Verification items for the finished model (mm, model axes). Face numbers are marked on the shaded views. Coordinates: 2 decimals unless noted, no trailing zeros. Order: outer loops, then holes, each group sorted by start corner. A loop starts at its lowest first (then second) coordinate and runs counter-clockwise, first axis right, second up. Notation, with made-up numbers: (53, 32.25) -> (104, 32.25) arc R18 cw to (104, 41.25) -> close; hole circle Ø11 at (77.5, 3.25). An arc over 180 degrees is marked (long way). Write item = value, one per line. Start each with the question number.
from build123d import *

# Parameters (mm, degrees)
SKETCH1_R           = 101.6
BOSS_EXTRUDE1_DEPTH = 76.2
SKETCH2_R           = 12.7
BOSS_EXTRUDE2_DEPTH = 609.6


with BuildPart() as part:
    # Sketch1 → Boss-Extrude1 (new body)
    with BuildSketch(Plane.XY):
        Circle(SKETCH1_R)
    boss_extrude1 = extrude(amount=BOSS_EXTRUDE1_DEPTH)

    # Sketch2 → Boss-Extrude2 (add)
    with BuildSketch(Plane.XY.offset(76.2)):
        Circle(SKETCH2_R)
    extrude(amount=BOSS_EXTRUDE2_DEPTH)

    # Mirror1: Boss-Extrude1 across plane
    add(boss_extrude1.mirror(Plane.XY.offset(381)))


solid = part.part
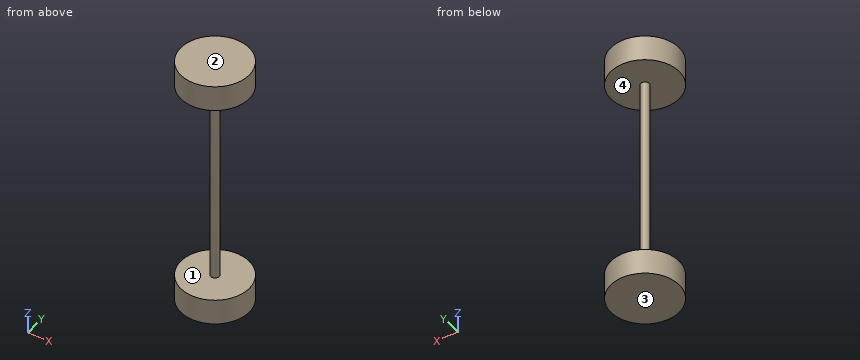
Item 1: Section check B-B (x = 73). Record the boundary of the cut face in (y, z), then the cut area to 3 significant figures.
Item 2: Gauge pin test, flat ends, axial feed: P1, Ø2, axis at y = 0, z = 361.5, coming from the -X side; P2, Ø12, axis at x = 1.5, z = 630, coming from the +Y side; P3, Ø3, axis at x = 50, y = 62.5, coming from the -Z side. Record the tip position at first contact, or that the pin passes through.
Item 3: Mould release check, pull along Z, two halves, no side actions. Record for the marked faces 1, 2, 3 and 4: pulls with the +Z half, pulls with the -Z half, needs draft (parallel to the pull), parting line crosses it, or undercut.
Item 4: Section check C-C (y = -37.5). Record the boundary of the cut face in (x, z), then the cut area to 3 significant figures.
Item 5: Section check A-A (y = 0). Record the boundary of the cut face in (x, z).
Item 6: Thickness scan on line 1 (Z direction, x = 6, y = 33.5); line 2 (X direction, y = 0.5, z = 121.5); line 3 (Y direction, x = -24.5, z = 708). Record the ranges inside material, lowest first.
Filled sheet:
q1.outline = (-70.67, 0) -> (70.67, 0) -> (70.67, 76.2) -> (-70.67, 76.2) -> close; (-70.67, 685.8) -> (70.67, 685.8) -> (70.67, 762) -> (-70.67, 762) -> close
q1.area = 21,500 mm^2
q2.P1 = -12.7
q2.P2 = 12.7
q2.P3 = 0
q3.face_1 = undercut
q3.face_2 = pulls with the +Z half
q3.face_3 = pulls with the -Z half
q3.face_4 = undercut
q4.outline = (-94.43, 0) -> (94.43, 0) -> (94.43, 76.2) -> (-94.43, 76.2) -> close; (-94.43, 685.8) -> (94.43, 685.8) -> (94.43, 762) -> (-94.43, 762) -> close
q4.area = 28,800 mm^2
q5.outline = (-101.6, 0) -> (101.6, 0) -> (101.6, 76.2) -> (12.7, 76.2) -> (12.7, 685.8) -> (101.6, 685.8) -> (101.6, 762) -> (-101.6, 762) -> (-101.6, 685.8) -> (-12.7, 685.8) -> (-12.7, 76.2) -> (-101.6, 76.2) -> close
q6.line_1 = 0 to 76.2, 685.8 to 762
q6.line_2 = -12.69 to 12.69
q6.line_3 = -98.6 to 98.6
